Here's how the part is built. I have some questions about the finished solid (model axes, mm). Give positions to 0.01 mm unless a question says otherwise; leave off trailing zeros. Write each loop counter-clockwise with the first axis right and the second up, starting at its lowest first coordinate (ties: lowest second). Pieces come first, ordered by that corner, then holes. Notation, with made-up numbers: (49.25, 44) -> (64.25, 44) arc R10 ccw to (64.25, 63) -> close; hole circle Ø4 at (46, -32.5). An arc over 180 degrees is marked (long way). Use one line per item in the form item = value.
```python
from build123d import *

# Parameters (mm, degrees)
MODEL_R             = 1.5
BOSS_EXTRUDE1_DEPTH = 2.55


with BuildPart() as part:
    # Model → Boss-Extrude1 (new body)
    with BuildSketch(Plane.XY):
        with BuildLine():
            Line((-4, 8.512011392), (-4, 7.745966692))
            ThreePointArc((-4, 7.745966692), (-4.317541634, 5.245966692), (-5.25, 2.90473751))
            ThreePointArc((-5.25, 2.90473751), (0, -6), (5.25, 2.90473751))
            ThreePointArc((5.25, 2.90473751), (4.317541634, 5.245966692), (4, 7.745966692))
            Line((4, 7.745966692), (4, 8.785724032))
            Line((4, 8.785724032), (4, 160))
            ThreePointArc((4, 160), (0, 164), (-4, 160))
            Line((-4, 160), (-4, 8.512011392))
        make_face()
        Circle(MODEL_R, mode=Mode.SUBTRACT)
        with Locations((0, 160)):
            Circle(MODEL_R, mode=Mode.SUBTRACT)
    extrude(amount=BOSS_EXTRUDE1_DEPTH)


solid = part.part
```
Q1. I want a section at B-B, the plane y = 0. Write out the boundary of the cut face in (x, z).
Result set:
outline = (-6, 0) -> (-1.5, 0) -> (-1.5, 2.55) -> (-6, 2.55) -> close; (1.5, 0) -> (6, 0) -> (6, 2.55) -> (1.5, 2.55) -> close
Q2. Will these pins go through, and if not, where does the flat tip stop? pin 1 Ø1.3 at (y, z) = (110, 1) entering from -X; pin 2 Ø3.5 at (x, y) = (0, 160) entering from +Z; pin 3 Ø0.8 at (y, z) = (71, 1) entering from +X.
Result set:
pin_1 = -4
pin_2 = 2.55
pin_3 = 4
Q3. If I drill on line 1 along Y through (x, z) = (0, 1.8); line 2 along X through (y, z) = (160, 1.2); line 3 along Y through (x, z) = (1.25, 1.6), over which ranges is the centre line in solid material (lowest first)? Write a range as from..to.
Result set:
line_1 = -6..-1.5, 1.5..158.5, 161.5..164
line_2 = -4..-1.5, 1.5..4
line_3 = -5.87..-0.83, 0.83..159.17, 160.83..163.8
Q4. I want a section at A-A, the plane z = 0.9. Write out the boundary of the cut face in (x, y).
Result set:
outline = (-5.25, 2.9) arc R6 ccw (long way) to (5.25, 2.9) arc R10 cw to (4, 7.75) -> (4, 160) arc R4 ccw to (-4, 160) -> (-4, 7.75) arc R10 cw to start; hole circle Ø3 at (0, 0); hole circle Ø3 at (0, 160)
Q5. I want a section at D-D, the plane y = 145. Write out the boundary of the cut face in (x, z).
Result set:
outline = (-4, 0) -> (4, 0) -> (4, 2.55) -> (-4, 2.55) -> close
Q6. If we mould it in two halves opening along Y, with no side actions, what happens to faces 1 (the face through (-0.195, 161.487, 1.257)), 2 (the face through (-1.5, 0.07, 1.26)), 3 (the face through (0, 80, 0)), 4 (the face through (0, -6, 1))? For each: +Y half, -Y half, draft (parallel to the pull), parting line (faces both ways), or undercut.
Result set:
face_1 = undercut
face_2 = undercut
face_3 = draft
face_4 = parting line
Q7. I want a section at C-C, the plane x = 0. Write out the boundary of the cut face in (y, z).
Result set:
outline = (-6, 0) -> (-1.5, 0) -> (-1.5, 2.55) -> (-6, 2.55) -> close; (1.5, 0) -> (158.5, 0) -> (158.5, 2.55) -> (1.5, 2.55) -> close; (161.5, 0) -> (164, 0) -> (164, 2.55) -> (161.5, 2.55) -> close
